Design review of the part shown in the three views and the two pictorial views. Dimensions are in mm from the part's minimum x, y and z. A direction names the side the tool comes from. Coordinates: 2 decimals unless noted, no trailing zeros. Loops run counter-clockwise (first coordinate to the right, second up) from the corner with the lowest first, then second, coordinate; pieces in that order, holes last. Notation, with made-up numbers: (-30, -2) -> (-15, -2) arc R17 cw to (-15, 11) -> close; hole circle Ø4 at (17, 41). An arc over 180 degrees is marked (long way). One line per item, written item: value. Start each with the question number.
1. Add section D-D on z = 10.5. Write out the cut boundary in (x, y).
2. Add section A-A on z = 60. Write out the cut boundary in (x, y), plus the area to 3 significant figures.
3. Draft analysis for pull direction Z (two halves, no side actions). For the marked faces 1 and 2, state which applies: pulls with the +Z half, pulls with the -Z half, needs draft (parallel to the pull), parting line crosses it, or undercut.
4. Add section C-C on x = 123. Write out the cut boundary in (y, z), plus the area to 3 significant figures.
5. Machinability: for the marked faces 3, 4 and 5, which of the approach directions +Z, -Z, +X, -X, +Y, -Y give a long, thin tool a straight path to every point of the face, cutting with its end or side? Answer none if there is none.
6. Add section B-B on x = 100. Write out the cut boundary in (y, z).
7. For probe 1 along Z at (x, y) = (71, 11.25); probe 2 along Z at (x, y) = (100, 17); probe 3 along X at (y, z) = (13.5, 60), list the stretches that pass through material, from the lowest coordinate up.
8. Insertion check: pin 1 (20.5 mm diameter, centred on x = 131.5, z = 112, fed in from +Y); pin 2 (7.5 mm diameter, centred on x = 109.5, z = 85, fed in from +Y); pin 3 (6 mm diameter, centred on x = 100, z = 60, fed in from -Y); pin 4 (12 mm diameter, centred on x = 78.5, z = 78, fed in from -Y). Each pin has a flat end and moves straight along its axis. Give the tip position at first contact, or say it passes through.
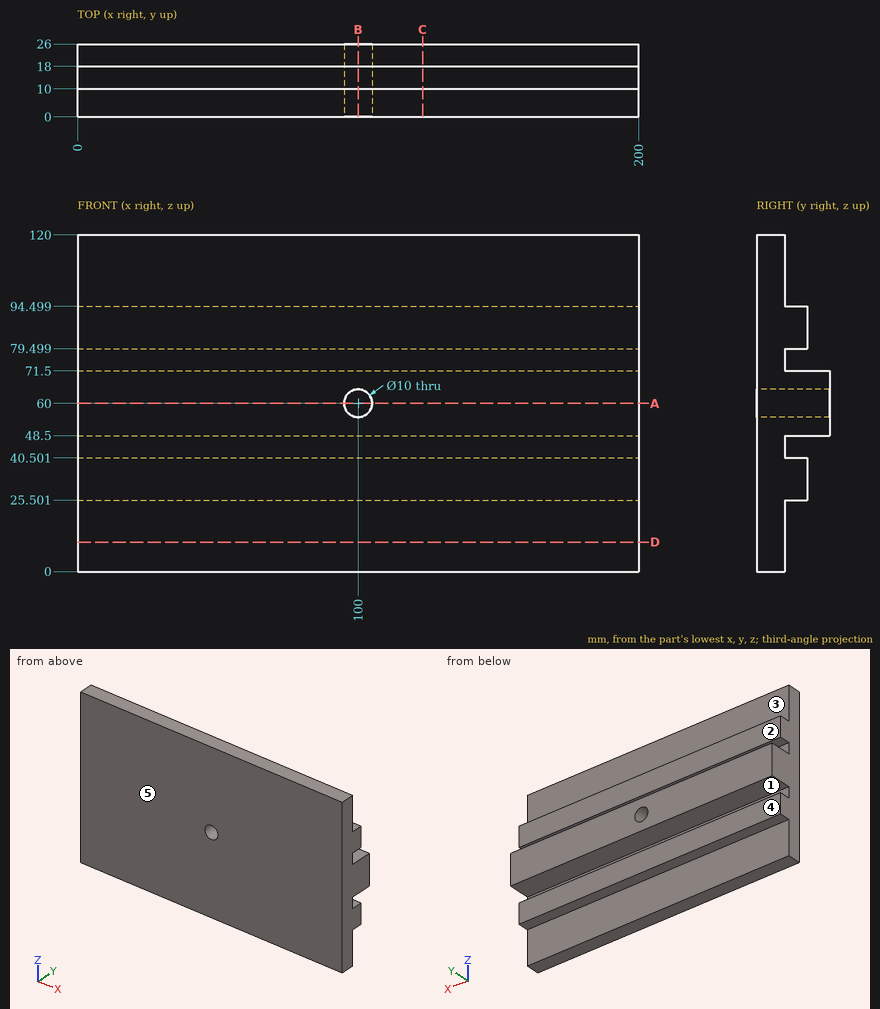
Worked answers:
1. outline: (0, 0) -> (200, 0) -> (200, 10) -> (0, 10) -> close
2. outline: (0, 0) -> (95, 0) -> (95, 26) -> (0, 26) -> close; (105, 0) -> (200, 0) -> (200, 26) -> (105, 26) -> close
2. area: 4,940 mm²
3. face 1: undercut
3. face 2: needs draft
4. outline: (0, 0) -> (10, 0) -> (10, 25.5) -> (18, 25.5) -> (18, 40.5) -> (10, 40.5) -> (10, 48.5) -> (26, 48.5) -> (26, 71.5) -> (10, 71.5) -> (10, 79.5) -> (18, 79.5) -> (18, 94.5) -> (10, 94.5) -> (10, 120) -> (0, 120) -> close
4. area: 1,810 mm²
5. face 3: +Z, +X, -X, +Y
5. face 4: -Z, +X, -X, +Y
5. face 5: +Z, -Z, +X, -X, -Y
6. outline: (0, 0) -> (10, 0) -> (10, 25.5) -> (18, 25.5) -> (18, 40.5) -> (10, 40.5) -> (10, 48.5) -> (26, 48.5) -> (26, 55) -> (0, 55) -> close; (0, 65) -> (26, 65) -> (26, 71.5) -> (10, 71.5) -> (10, 79.5) -> (18, 79.5) -> (18, 94.5) -> (10, 94.5) -> (10, 120) -> (0, 120) -> close
7. probe 1: z = 25.5 to 40.5, 48.5 to 71.5, 79.5 to 94.5
7. probe 2: z = 25.5 to 40.5, 48.5 to 55, 65 to 71.5, 79.5 to 94.5
7. probe 3: x = 0 to 95, 105 to 200
8. pin 1: stops at y = 10
8. pin 2: stops at y = 18
8. pin 3: passes through
8. pin 4: stops at y = 0
